```python
from build123d import *

# Parameters (mm, degrees)
SKETCH_1_W      = 90
SKETCH_1_H      = 4
EXTRUDE_1_DEPTH = 24
SKETCH_2_W      = 90
SKETCH_2_H      = 4
EXTRUDE_2_DEPTH = 24
SKETCH_3_W      = 90
SKETCH_3_H      = 66
EXTRUDE_3_DEPTH = 24


with BuildPart() as part:
    # Sketch 1 → Extrude 1 (new body)
    with BuildSketch(Plane.XY):
        with Locations((0, 31)):
            Rectangle(SKETCH_1_W, SKETCH_1_H)
    extrude(amount=EXTRUDE_1_DEPTH)



with BuildPart() as body_2:
    # Sketch 2 → Extrude 2 (new body)
    with BuildSketch(Plane.XY):
        with Locations((0, -31)):
            Rectangle(SKETCH_2_W, SKETCH_2_H)
    extrude(amount=EXTRUDE_2_DEPTH)


with BuildPart() as part_1:
    add(part.part)

    add(body_2.part)  # Extrude 3 merges body 2
    # Sketch 3 → Extrude 3 (add)
    with BuildSketch(Plane.XY.offset(24)):
        Rectangle(SKETCH_3_W, SKETCH_3_H)
    extrude(amount=EXTRUDE_3_DEPTH)


solid = part_1.part
```
Here's how the part is built. I have some questions about the finished solid (model axes, mm). A direction names the side the tool comes from. Round coordinates to 2 decimals unless told otherwise and drop trailing zeros. Order: outer loops, then holes, each group sorted by start corner. A loop starts at its lowest first (then second) coordinate and runs counter-clockwise, first axis right, second up. Notation, with made-up numbers: M 84,47 L 105,47 A17 cw 105,70 Z; hole C -28,6.25 d7. An arc over 180 degrees is marked long. Use CSV: the item, a comma, the result in double quotes.
1) I want a section at C-C (y = -20.5). List the corners of the cut face in (x, z) for me, then the cut area to 3 significant figures.
Taken from the geometry:
outline,"M -45,24 L 45,24 L 45,48 L -45,48 Z"
area,"2,160 mm^2"
2) I'm going to push a flat-ended pin straight in: P1, Ø1, axis at x = 6.5, y = 6.5, coming from the -Z side. Where does the tip first touch, or does it pass through?
Taken from the geometry:
P1,"z = 24"
3) I need wall thicknesses on line 1 along Y through (x, z) = (-18.5, 9); line 2 along Z through (x, y) = (27.5, -6). Which ranges of each line are inside material? Lowest first, please. Write a range as [from, to].
Taken from the geometry:
line 1,"[-33, -29], [29, 33]"
line 2,"[24, 48]"
4) On a 3-axis mill with a long thin cutter (end or side, diameter ignored), from which of +Z, -Z, +X, -X, +Y, -Y can I reach the whole of each face in a straight line? I mean faces 4 (the flat face through (-1, 33, 24)), 5 (the flat face through (-1, -29, 12)). Say none if no direction works.
Taken from the geometry:
face 4,"+Z, -Z, +X, -X, +Y"
face 5,"-Z, +X, -X"
5) I want a section at A-A (z = 22). List the corners of the cut face in (x, y) for me.
Taken from the geometry:
outline,"M -45,-33 L 45,-33 L 45,-29 L -45,-29 Z; M -45,29 L 45,29 L 45,33 L -45,33 Z"
6) If we mould it in two halves opening along Y, with no side actions, what happens to faces 1 (the flat face through (-1, -31, 0)), 2 (the flat face through (-1, -33, 24)), 3 (the flat face through (-1, 29, 12))? For each: pulls with the +Y half, pulls with the -Y half, needs draft (parallel to the pull), parting line crosses it, or undercut.
Taken from the geometry:
face 1,"needs draft"
face 2,"pulls with the -Y half"
face 3,"undercut"
7) I want a section at B-B (x = -24). List the corners of the cut face in (y, z) for me, then the cut area to 3 significant figures.
Taken from the geometry:
outline,"M -33,0 L -29,0 L -29,24 L 29,24 L 29,0 L 33,0 L 33,48 L -33,48 Z"
area,"1,780 mm^2"
